Part model, mm, in its own coordinate system. A direction names the side the tool comes from. Round coordinates to 2 decimals unless told otherwise and drop trailing zeros. Loops run counter-clockwise (first coordinate to the right, second up) from the corner with the lowest first, then second, coordinate; pieces in that order, holes last.
1) Band-saw the part on C-C, the plane z = 73. Write the cut outline in (x, y), then the cut area to 3 significant figures.
2) 3-axis set-ups, long thin cutter, end or side, ignore diameter. For faces 5 (the flat face through (2.028, 53.718, 36.333)), 6 (the flat face through (2, 76, 2)), 7 (the flat face through (2, 47, 156)), 8 (the flat face through (2, 4, 140)): which of +Z, -Z, +X, -X, +Y, -Y reach the whole face in a straight line?
3) Band-saw the part on A-A, the plane y = 39. Write the cut outline in (x, z), then the cut area to 3 significant figures.
4) Band-saw the part on B-B, the plane z = 96.5. Write the cut outline in (x, y), then the cut area to 3 significant figures.
5) Drop flat-ended pins along their axis: P1, Ø1.2, axis at x = 2.5, z = 97, coming from the -Y side; P2, Ø1.2, axis at x = 2.5, y = 78, coming from the -Z side; P3, Ø2, axis at x = 3, y = 4.5, coming from the -Z side. Give the stop position or say it passes through.
6) Probe line 1 (Z direction, x = 2.8, y = 5); line 2 (Z direction, x = 0.25, y = 6); line 3 (Y direction, x = 3.15, z = 77). List the from-to ranges inside material, lowest first.
7) Mould opens along Z. For faces 1 (the cylindrical face through (2.028, 7.736, 147.639)), 2 (the cylindrical face through (2.03, 1.75, 145.09)), 3 (the cylindrical face through (2.028, 14.014, 10.703)), 4 (the flat face through (2, 80, 2)) say: +Z half, -Z half, draft (parallel to the pull), parting line (faces both ways), or undercut.
8) Band-saw the part on D-D, the plane x = 3.2. State how many separate pieces and enclosed holes the cut face has, then the cut area to 3 significant figures.
from build123d import *

# Parameters (mm, degrees)
F0_W      = 96
F0_H      = 160
F1_DEPTH  = 4
F2_W      = 4
F2_H      = 5
F2_W_2    = 88
F2_H_2    = 4
F3_DEPTH  = 4
F5_DEPTH  = 4
F7_DEPTH  = 4
F9_DEPTH  = 4.001
F11_DEPTH = 4


with BuildPart() as f1:
    # F0 (on Right) → F1 (new body)
    with BuildSketch(Plane.YZ):
        with Locations((48, 80)):
            Rectangle(F0_W, F0_H)
    extrude(amount=F1_DEPTH)

    # F2 (on face) → F3 (cut, through all)
    with BuildSketch(Plane.YZ.offset(4)):
        with Locations((78, 2.5)):
            Rectangle(F2_W, F2_H)
        with Locations((48, 158)):
            Rectangle(F2_W_2, F2_H_2)
    extrude(amount=-F3_DEPTH, mode=Mode.SUBTRACT)

    # F4 (on face) → F5 (cut, through all)
    with BuildSketch(Plane.YZ.offset(4)):
        Polygon((54.719311, 88.064946), (57, 91.351046), (14.280689, 121), (12, 117.713899), align=None)
        Polygon((89.066517, 60.420493), (15.531596, 19.817348), (17.465079, 16.315685), (91, 56.91883), align=None)
    extrude(amount=-F5_DEPTH, mode=Mode.SUBTRACT)

    # F6 (on face) → F7 (cut, through all)
    with BuildSketch(Plane.YZ.offset(4)):
        with BuildLine():
            Line((0, 140), (0, 0))
            Line((0, 0), (28, 0))
            Line((28, 0), (28, 5))
            ThreePointArc((28, 5), (13.857864, 10.857864), (8, 25))
            Line((8, 25), (8, 140))
            Line((8, 140), (0, 140))
        make_face()
    extrude(amount=-F7_DEPTH, mode=Mode.SUBTRACT)

    # F8 (on face) → F9 (cut, through all)
    with BuildSketch(Plane.YZ.offset(4)):
        with BuildLine():
            ThreePointArc((6.07792, 141.933962), (7.712282, 142.357475), (9.394599, 142.5))
            Line((9.394599, 142.5), (90.076656, 142.5))
            ThreePointArc((90.076656, 142.5), (92.804022, 147.25), (90.076656, 152))
            Line((90.076656, 152), (60.076656, 152))
            Line((60.076656, 152), (60.076656, 150))
            ThreePointArc((60.076656, 150), (60.369549, 149.292893), (61.076656, 149))
            Line((61.076656, 149), (81.576656, 149))
            ThreePointArc((81.576656, 149), (82.637316, 146.43934), (80.076656, 147.5))
            Line((80.076656, 147.5), (9.394599, 147.5))
            ThreePointArc((9.394599, 147.5), (7.712282, 147.642525), (6.07792, 148.066038))
            ThreePointArc((6.07792, 148.066038), (1.75, 145), (6.07792, 141.933962))
        make_face()
    extrude(amount=-F9_DEPTH, mode=Mode.SUBTRACT)

    # F10 (on face) → F11 (cut, through all)
    with BuildSketch(Plane.YZ.offset(4)):
        with BuildLine():
            ThreePointArc((9.411765, 134.352941), (10.910428, 137.727607), (8, 140))
            Line((8, 140), (8, 132))
            ThreePointArc((8, 132), (8.380019, 133.371989), (9.411765, 134.352941))
        make_face()
    extrude(amount=-F11_DEPTH, mode=Mode.SUBTRACT)


solid = f1.part
Reported:
1. outline: (0, 8) - (4, 8) - (4, 96) - (0, 96) - close
1. area: 352 mm2
2. face 5: +X, -X
2. face 6: -Z, +X, -X
2. face 7: +Z, +X, -X
2. face 8: -Z, +X, -X, -Y
3. outline: (0, 0) - (4, 0) - (4, 28.21) - (0, 28.21) - close; (0, 32.78) - (4, 32.78) - (4, 98.97) - (0, 98.97) - close; (0, 103.84) - (4, 103.84) - (4, 142.5) - (0, 142.5) - close; (0, 147.5) - (4, 147.5) - (4, 156) - (0, 156) - close
3. area: 566 mm2
4. outline: (0, 8) - (4, 8) - (4, 42.57) - (0, 42.57) - close; (0, 49.58) - (4, 49.58) - (4, 96) - (0, 96) - close
4. area: 324 mm2
5. P1: stops at y = 8
5. P2: stops at z = 5
5. P3: stops at z = 140
6. line 1: z = 140 to 141.75, 148.25 to 156
6. line 2: z = 140 to 141.91, 148.09 to 156
6. line 3: y = 8 to 96
7. face 1: undercut
7. face 2: undercut
7. face 3: -Z half
7. face 4: draft
8. separate pieces: 1
8. enclosed holes: 3
8. area: 12,600 mm2
